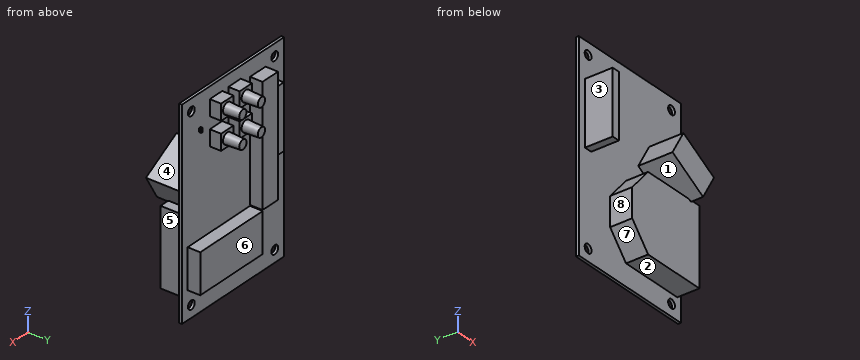
```python
from build123d import *

# Parameters (mm, degrees)
SKETCH1_W                           = 41.91
SKETCH1_H                           = 64.77
BOARD_DEPTH                         = 0.9144
BUTTONBASE_W                        = 5.08
BUTTONBASE_H                        = 5.08
BUTTON_DEPTH                        = 3.6068
SKETCH4_W                           = 25.654
SKETCH4_H                           = 12.7
LIPO_DEPTH                          = 4.064
F_7_64_0_10938_DIAMETER_HOLE1_D     = 2.778252
F_7_64_0_10938_DIAMETER_HOLE1_DEPTH = 25.4
F_7_64_0_10938_DIAMETER_HOLE1_TIP   = 0.834671108
SKETCH8_W                           = 0.635
SKETCH8_H                           = 1.27
LED_DEPTH                           = 0.635
POWERJACK_DEPTH                     = 10.9982
XBEE_DEPTH                          = 7.09
SKETCH12_R                          = 1.7526
BUTTONPLUNGER_DEPTH                 = 5
PLUNGER_TAPER_ANGLE                 = 2.87
SKETCH13_W                          = 6.35
SKETCH13_H                          = 37.846
ATMEL_DEPTH                         = 4
HEADERS_DEPTH                       = 8.89
HEADERS_DEPTH_BACK                  = 2.8194
SKETCH15_W                          = 2.54
SKETCH15_H                          = 20.32


with BuildPart() as part:
    # Sketch1 → Board (new body)
    with BuildSketch(Plane(origin=(0, 0, 0), x_dir=(1, 0, 0), z_dir=(0, 1, 0))):
        with Locations((20.955, 32.385)):
            Rectangle(SKETCH1_W, SKETCH1_H)
    extrude(amount=BOARD_DEPTH)

    # ButtonBase → Button (add)
    with BuildSketch(Plane(origin=(0, 0.9144, 0), x_dir=(1, 0, 0), z_dir=(0, 1, 0))):
        with Locations((20.32, 15.24)):
            Rectangle(BUTTONBASE_W, BUTTONBASE_H)
        with Locations((27.94, 15.24)):
            Rectangle(BUTTONBASE_W, BUTTONBASE_H)
        with Locations((27.94, 6.35)):
            Rectangle(BUTTONBASE_W, BUTTONBASE_H)
        with Locations((20.32, 6.35)):
            Rectangle(BUTTONBASE_W, BUTTONBASE_H)
    extrude(amount=BUTTON_DEPTH)

    # Sketch4 → LiPo (add)
    with BuildSketch(Plane(origin=(0, 0.9144, 0), x_dir=(1, 0, 0), z_dir=(0, 1, 0))):
        with Locations((26.797, 49.53)):
            Rectangle(SKETCH4_W, SKETCH4_H)
    extrude(amount=LIPO_DEPTH)

    # 7/64 (0.10938) Diameter Hole1
    with Locations(Plane(origin=(0, 0.9144, 0), x_dir=(1, 0, 0), z_dir=(0, 1, 0))):
        with Locations((3.81, 60.96), (38.1, 60.96), (38.1, 3.81), (3.81, 3.81)):
            Hole(F_7_64_0_10938_DIAMETER_HOLE1_D / 2, depth=F_7_64_0_10938_DIAMETER_HOLE1_DEPTH)
            with Locations((0, 0, -(F_7_64_0_10938_DIAMETER_HOLE1_DEPTH + F_7_64_0_10938_DIAMETER_HOLE1_TIP / 2))):  # 118° drill point
                Cone(0, F_7_64_0_10938_DIAMETER_HOLE1_D / 2, F_7_64_0_10938_DIAMETER_HOLE1_TIP, mode=Mode.SUBTRACT)

    # Sketch8 → LED (add)
    with BuildSketch(Plane(origin=(0, 0.9144, 0), x_dir=(1, 0, 0), z_dir=(0, 1, 0))):
        with Locations((34.544, 10.8585)):
            Rectangle(SKETCH8_W, SKETCH8_H)
    extrude(amount=LED_DEPTH)

    # Sketch10 → PowerJack (add)
    with BuildSketch(Plane.XZ):
        Polygon((41.478212841, -26.21822299), (28.9179, -18.96652299), (24.4221, -26.75347701), (36.982412841, -34.00517701), align=None)
    extrude(amount=POWERJACK_DEPTH)

    # Sketch11 → XBee (add)
    with BuildSketch(Plane.XZ):
        Polygon((19.3929, -57.912), (12.8651, -50.3174), (12.8651, -41.1226), (19.3929, -33.528), (40.4749, -33.528), (40.4749, -57.912), align=None)
    extrude(amount=XBEE_DEPTH)

    # Sketch12 → ButtonPlunger (add)
    with BuildSketch(Plane(origin=(0, 4.5212, 0), x_dir=(1, 0, 0), z_dir=(0, 1, 0))):
        with Locations(Location((20.32, 15.24, 0), (0, 0, 90))):
            Circle(SKETCH12_R)
        with Locations(Location((27.94, 15.24, 0), (0, 0, 270))):
            Circle(SKETCH12_R)
        with Locations(Location((27.94, 6.35, 0), (0, 0, 270))):
            Circle(SKETCH12_R)
        with Locations(Location((20.32, 6.35, 0), (0, 0, 270))):
            Circle(SKETCH12_R)
    extrude(amount=BUTTONPLUNGER_DEPTH)

    # Plunger Taper
    plunger_taper_faces = [part.faces().sort_by_distance(p)[0] for p in [
        (27.94, 7.0212, -8.1026),
        (27.94, 7.0212, -16.9926),
        (20.32, 7.0212, -13.4874),
        (20.32, 7.0212, -8.1026),
    ]]
    draft(plunger_taper_faces, Plane.ZX.offset(4.5212), PLUNGER_TAPER_ANGLE)

    # Sketch13 → ATMEL (add)
    with BuildSketch(Plane(origin=(0, 0.9144, 0), x_dir=(1, 0, 0), z_dir=(0, 1, 0))):
        with Locations((10.795, 24.003)):
            Rectangle(SKETCH13_W, SKETCH13_H)
    extrude(amount=ATMEL_DEPTH)

    # Sketch15 → Headers (add, two sides: drawn at the far end of the back side and taken through both)
    with BuildSketch(Plane(origin=(0, 0, 0), x_dir=(-1, 0, 0), z_dir=(0, -1, 0)).offset(-HEADERS_DEPTH_BACK)):
        with Locations((-3.81, 21.59)):
            Rectangle(SKETCH15_W, SKETCH15_H)
    extrude(amount=HEADERS_DEPTH + HEADERS_DEPTH_BACK)


solid = part.part
```
Can you work these out from the model? Positions are in its coordinate system, mm. Face numbers are marked on the shaded views. A direction names the side the tool comes from. Round coordinates to 2 decimals unless told otherwise and drop trailing zeros. Order: outer loops, then holes, each group sorted by start corner. A loop starts at its lowest first (then second) coordinate and runs counter-clockwise, first axis right, second up. Notation, with made-up numbers: (21, 22.5) -> (29, 22.5) arc R11 cw to (29, 40.5) -> close; hole circle Ø9 at (15, 79). An arc over 180 degrees is marked (long way). Return JSON: item names as keys, results as strings. Group by question number.
1. I need wall thicknesses on line 1 (Z direction, x = 3.81, y = 0.4); line 2 (X direction, y = 0.6, z = -60.96); line 3 (Y direction, x = 10.5, z = -48.5). Which ranges of each line are inside material? Lowest first, please. Write a range as [from, to].
2. We'd pull the mould along X, two halves only. Please class the marked faces 1, 2 and 3: released by +X, released by -X, zero draft, split by the parting line, or undercut.
3. If we section it at D-D, the plane x = 20.32: Write out the boundary of the cut face in (y, z).
4. If we section it at A-A, the plane x = 3.81: Write out the boundary of the cut face in (y, z), then the cut area to 4 significant figures.
5. Will these pins go through, and if not, where does the flat tip stop? pin 1 (8 mm diameter, centred on x = 30, z = -56, fed in from -Y); pin 2 (3 mm diameter, centred on x = 20, y = 3, fed in from -Z); pin 3 (0.8 mm diameter, centred on x = 4, z = -19.5, fed in from -Y); pin 4 (1 mm diameter, centred on y = -1, z = -7.5, fed in from -X).
6. Which directions (+Z, -Z, +X, -X, +Y, -Y) give clear straight access to the entire face, cutting with the end or side of a thin tool? Please do the marked faces 4, 5, 6, 7 and 8.
7. If we section it at B-B, the plane y = -3.75: Write out the boundary of the cut face in (x, z), then the cut area to 3 significant figures.
Output values:
{
 "1": {"line 1": "[-64.77, -62.35], [-59.57, -5.2], [-2.42, 0]", "line 2": "[0, 2.42], [5.2, 36.71], [39.49, 41.91]", "line 3": "[0, 0.91]"},
 "2": {"face 1": "undercut", "face 2": "zero draft", "face 3": "released by -X"},
 "3": {"outline": "(-7.09, -57.91) -> (0, -57.91) -> (0, -64.77) -> (0.91, -64.77) -> (0.91, -55.88) -> (4.98, -55.88) -> (4.98, -43.18) -> (0.91, -43.18) -> (0.91, -17.78) -> (4.52, -17.78) -> (4.52, -16.99) -> (9.52, -16.74) -> (9.52, -13.74) -> (4.52, -13.49) -> (4.52, -12.7) -> (0.91, -12.7) -> (0.91, -8.89) -> (4.52, -8.89) -> (4.52, -8.1) -> (9.52, -7.85) -> (9.52, -4.85) -> (4.52, -4.6) -> (4.52, -3.81) -> (0.91, -3.81) -> (0.91, 0) -> (0, 0) -> (0, -33.53) -> (-7.09, -33.53) -> close"},
 "4": {"outline": "(-8.89, -31.75) -> (0, -31.75) -> (0, -59.57) -> (0.91, -59.57) -> (0.91, -31.75) -> (2.82, -31.75) -> (2.82, -11.43) -> (0.91, -11.43) -> (0.91, -5.2) -> (0, -5.2) -> (0, -11.43) -> (-8.89, -11.43) -> close; (0, -64.77) -> (0.91, -64.77) -> (0.91, -62.35) -> (0, -62.35) -> close; (0, -2.42) -> (0.91, -2.42) -> (0.91, 0) -> (0, 0) -> close", "area": "273.5 mm²"},
 "5": {"pin 1": "y = -7.09", "pin 2": "z = -55.88", "pin 3": "y = -8.89", "pin 4": "through"},
 "6": {"face 4": "+Z, +X, -Y", "face 5": "-Z, +X, -Y", "face 6": "-Z, +X, -X, +Y", "face 7": "-Z, -X, -Y", "face 8": "+Z, -Z, -X, -Y"},
 "7": {"outline": "(2.54, -31.75) -> (5.08, -31.75) -> (5.08, -11.43) -> (2.54, -11.43) -> close; (12.87, -50.32) -> (19.39, -57.91) -> (40.47, -57.91) -> (40.47, -33.53) -> (37.26, -33.53) -> (41.48, -26.22) -> (28.92, -18.97) -> (24.42, -26.75) -> (36.16, -33.53) -> (19.39, -33.53) -> (12.87, -41.12) -> close", "area": "805 mm²"}
}
